Check sheet for the modelled part. Datum: model origin and axes. Units: mm. A direction names the side the tool comes from. Round coordinates to 2 decimals unless told otherwise and drop trailing zeros. Write each loop counter-clockwise with the first axis right and the second up, starting at its lowest first coordinate (ties: lowest second). Pieces come first, ordered by that corner, then holes. Notation, with made-up numbers: M 88.25,-29 L 123.25,-29 A36 ccw 123.25,8 Z; hole C 82.25,-30.5 d7. An arc over 180 degrees is marked long. Answer in a Markdown table with one row per item.
Autodesk Inventor part; units mm, degrees
ref_plane "Cross Section Plane" through (9.3224, -14.1105, 0) normal (0.9904, -0.1379, 0) x (0, 0, 1)
ref_plane "Work Plane2" through (9.981, -9.3815, 0) normal (-1, 0, 0) x (0, 0, 1)
ref_plane "Work Plane3" through (79.2105, -9.3815, 0) normal (-0.9998, -0.0189, 0) x (0, 0, 1)
sketch "Sketch Path" plane through (0, 0, 0) normal (0, 0, 1) x (1, 0, 0)
  arc A0 (9.936, -4.607) -> (9.3224, -14.1105) centre (9.981, -9.3815) ccw
  arc A1 (28.5872, -4.4313) -> (29.4465, -4.3455) centre (28.542, 0.3685) ccw
  arc A2 (77.2347, -23.5685) -> (76.5111, 4.6858) centre (79.2105, -9.3815) ccw
  line L0 (77.2347, -23.5685) -> (9.3224, -14.1105)
  line L1 (9.936, -4.607) -> (28.5872, -4.4313)
  line L2 (29.4465, -4.3455) -> (76.5111, 4.6858)
ref_plane "Cross Section Plane" through (9.3224, -14.1105, 0) normal (0.9904, -0.1379, 0) x (0, 0, 1)
ref_plane "Work Plane2" through (9.981, -9.3815, 0) normal (-1, 0, 0) x (0, 0, 1)
ref_plane "Work Plane3" through (79.2105, -9.3815, 0) normal (-0.9998, -0.0189, 0) x (0, 0, 1)
sketch "Cross Section" plane through (9.3224, -14.1105, 0) normal (0.9904, -0.1379, 0) x (0, 0, 1)
  line L0 (-2, 0.3) -> (2, 0.3)
  line L1 (2, 0.3) -> (2, -0.3)
  line L2 (2, -0.3) -> (-2, -0.3)
  line L3 (-2, -0.3) -> (-2, 0.3)
  line L4 (-2, 0) -> (2, 0) construction
  point P0 (0, 0)
  point P1 (0, 0)
  dimension "d0" = 4
  dimension "d4" = 0.3
  dimension "d5" = 0.3
sweep "Belt" add profiles "Cross Section" path "Sketch Path"
equation "\"d0\" = da_B"
equation "\"d4\" = da_a"
equation "\"d5\" = da_a2"
equation "\"da_B\" = 4"
equation "\"da_pb\" = 2.5"
equation "\"da_a\" = 0.3"
equation "\"da_S\" = 1.5"
equation "\"da_Beta\" = 20deg"
equation "\"da_Ht\" = 0.7"
equation "\"da_H\" = 1.3"
equation "\"da_a2\" = 0.3"
properties part number "Synchronous Belt" material "Rubber"
1. Scan lines: L1, parallel to Y at x = 9, z = 1.1; L2, parallel to X at y = -10, z = -0.7; L3, parallel to X at y = -12.5, z = 0.7. Record each from-to range of solid material in increasing order.
Found:
| item | result |
|---|---|
| L1 | y = -14.36 to -13.75, -5.02 to -4.4 |
| L2 | x = 4.94 to 5.55, 93.22 to 93.82 |
| L3 | x = 5.98 to 6.77, 92.88 to 93.5 |
2. Access from +Z, -Z, +X, -X, +Y, -Y to the whole of each face (thin tool, end or side, straight path). Record for faces 4 (the face through (43.8, -18.61, -0.03)), 5 (the face through (52, 0, -2)).
Found:
| item | result |
|---|---|
| face 4 | +Z, -Z |
| face 5 | -Z, +X, -X, +Y, -Y |
3. Section check B-B, the plane y = -21.25. Record the cut outline in (x, z), and give its area (3 significant figures).
Found:
| item | result |
|---|---|
| outline | M 58.41,-2 L 62.76,-2 L 62.76,2 L 58.41,2 Z; M 86.68,-2 L 87.75,-2 L 87.75,2 L 86.68,2 Z |
| area | 21.7 mm2 |
4. Section check C-C, the plane x = 87.5. Record the cut outline in (y, z).
Found:
| item | result |
|---|---|
| outline | M -21.43,-2 L -20.69,-2 L -20.69,2 L -21.43,2 Z; M 1.93,-2 L 2.67,-2 L 2.67,2 L 1.93,2 Z |
5. Go/stop test with flat-tipped pins: pin 1 (2 mm diameter, centred on y = -12.5, z = 0, fed in from +X); pin 2 (2 mm diameter, centred on x = 71.5, z = -0.5, fed in from -Y). Record where each tip stops, or that it passes through.
Found:
| item | result |
|---|---|
| pin 1 | stops at x = 93.68 |
| pin 2 | stops at y = -23.21 |
6. Section check A-A, the plane z = 0.6. Record the cut outline in (x, y), and give its area (3 significant figures).
Found:
| item | result |
|---|---|
| outline | M 9.28,-14.41 L 77.19,-23.87 A14.62 ccw long 76.45,4.98 L 29.39,-4.05 A4.5 cw 28.58,-4.13 L 9.93,-4.31 A5.07 ccw Z; hole M 9.36,-13.81 L 77.28,-23.27 A14.02 ccw long 76.57,4.39 L 29.5,-4.64 A5.1 cw 28.59,-4.73 L 9.94,-4.91 A4.47 ccw Z |
| area | 120 mm2 |
7. Draft check along Y on faces 1 (the face through (56.4, 0.8, 2)), 2 (the face through (52.59, 0.4, 0.03)), 3 (the face through (52.706, -0.188, -0.028)). Enter one of: +Y half, -Y half, draft (parallel to the pull), parting line (faces both ways), or undercut.
Found:
| item | result |
|---|---|
| face 1 | draft |
| face 2 | +Y half |
| face 3 | undercut |
